Geometry check sheet. Reference: drawing and pictorial views, mm from the part's lowest x, y, z. A direction names the side the tool comes from. Coordinates: 2 decimals unless noted, no trailing zeros. Loops run counter-clockwise (first coordinate to the right, second up) from the corner with the lowest first, then second, coordinate; pieces in that order, holes last. Notation, with made-up numbers: (66.5, -9) - (93.5, -9) arc R11 ccw to (93.5, 1) - close; hole circle Ø3 at (53, -29.5). An arc over 180 degrees is marked (long way). One line per item, written item: value.
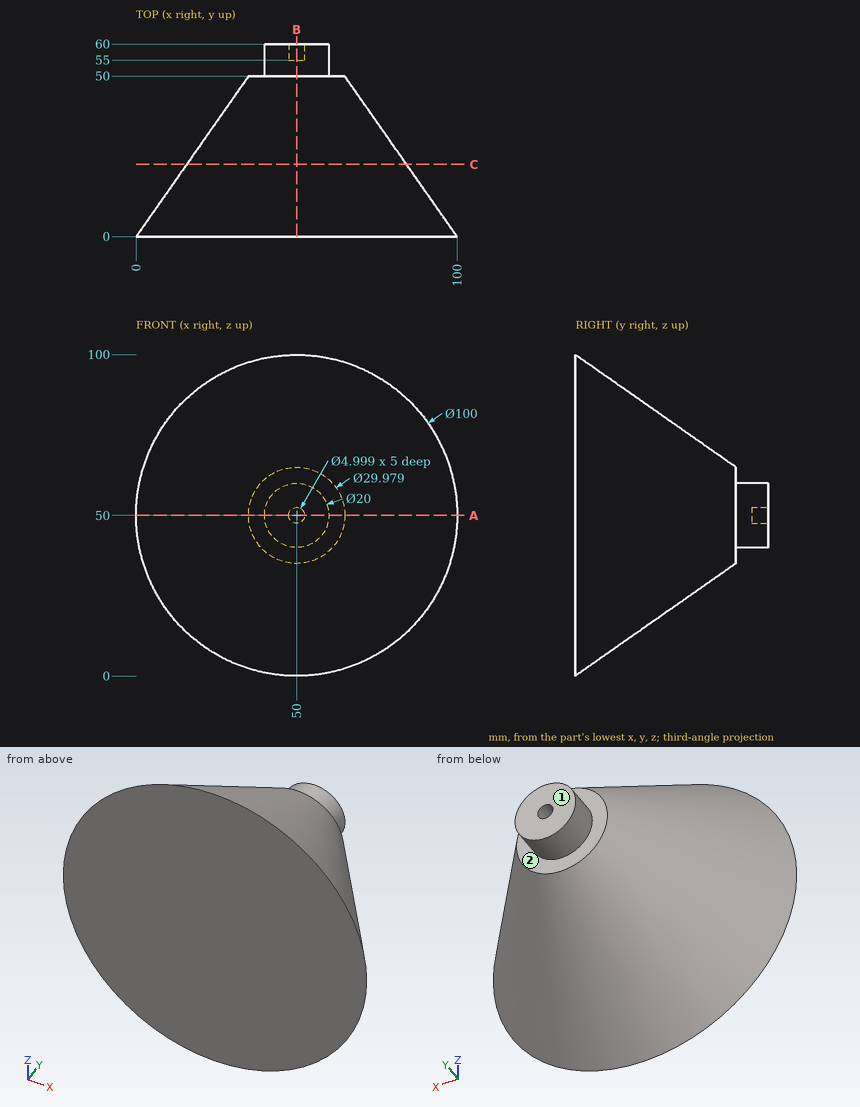
(1) Cross-section at B-B on x = 50. Record the cut outline in (y, z).
Reply:
outline: (0, 0) - (50, 35.01) - (50, 40) - (60, 40) - (60, 47.5) - (55, 47.5) - (55, 52.5) - (60, 52.5) - (60, 60) - (50, 60) - (50, 64.99) - (0, 100) - close
(2) Go/stop test with flat-tipped pins: pin 1 Ø2.5 at (x, z) = (50, 50) entering from +Y; pin 2 Ø6 at (x, y) = (28, 35.5) entering from -Z; pin 3 Ø8 at (x, y) = (78.5, 13) entering from +Z; pin 4 Ø1.5 at (x, z) = (87, 86) entering from -Y. Record where each tip stops, or that it passes through.
Reply:
pin 1: y = 55
pin 2: z = 32.28
pin 3: z = 84.36
pin 4: through
(3) Access from +Z, -Z, +X, -X, +Y, -Y to the whole of each face (thin tool, end or side, straight path). Record for the marked faces 1 and 2.
Reply:
face 1: +Z, -Z, +X, -X, +Y
face 2: +Y
(4) Cross-section at A-A on z = 50. Record the cut outline in (x, y).
Reply:
outline: (0, 0) - (100, 0) - (64.99, 50) - (60, 50) - (60, 60) - (52.5, 60) - (52.5, 55) - (47.5, 55) - (47.5, 60) - (40, 60) - (40, 50) - (35.01, 50) - close
(5) Cross-section at C-C on y = 22.5. Record the cut outline in (x, z) (1 decimal).
Reply:
outline: circle Ø68.5 at (50, 50)
(6) Material ranges on probe 1 along Z at (x, y) = (50, 58); probe 2 along Y at (x, z) = (44, 61); probe 3 along Y at (x, z) = (48, 16.5), recorded low to high. Write a range as from..to.
Reply:
probe 1: 40..47.5, 52.5..60
probe 2: 0..50
probe 3: 0..23.48
